Source: CAD feature listing. Evaluate the final solid. Frame: model axes, mm. Face numbers are marked on the shaded views. Coordinates: 2 decimals unless noted, no trailing zeros. Order: outer loops, then holes, each group sorted by start corner. A loop starts at its lowest first (then second) coordinate and runs counter-clockwise, first axis right, second up.
Autodesk Fusion 360 part; units mm, degrees
sketch "Sketch1" plane through (0, 0, 0) normal (0, 0, 1) x (1, 0, 0)
  line L0 (30, 30) -> (-30, 30)
  line L1 (-30, 30) -> (-30, -30)
  line L2 (-30, -30) -> (30, -30)
  line L3 (30, -30) -> (30, 30)
  line L4 (30, 30) -> (-30, -30) construction
  line L5 (-30, 30) -> (30, -30) construction
  circle A0 centre (-30, 30) radius 2.8
  circle A1 centre (30, 30) radius 2.8
  circle A2 centre (-30, -30) radius 2.8
  circle A3 centre (30, -30) radius 2.8
  line L6 (50, 50) -> (-50, 50)
  line L7 (-50, 50) -> (-50, -50)
  line L8 (-50, -50) -> (50, -50)
  line L9 (50, -50) -> (50, 50)
  line L10 (50, 50) -> (-50, -50) construction
  line L11 (-50, 50) -> (50, -50) construction
  line L12 (50, 50) -> (-50, 50)
  line L13 (-50, 50) -> (-50, 60)
  line L14 (-50, 60) -> (50, 60)
  line L15 (50, 60) -> (50, 50)
  line L16 (50, -50) -> (-50, -50)
  line L17 (-50, -50) -> (-50, -60)
  line L18 (-50, -60) -> (50, -60)
  line L19 (50, -60) -> (50, -50)
  circle A4 centre (-30, 30) radius 2
  circle A5 centre (30, 30) radius 2
  circle A6 centre (-30, -30) radius 2
  circle A7 centre (30, -30) radius 2
  dimension "d1" = 60
  dimension "d2" = 60
  dimension "d3" = 5.6
  dimension "d6" = 60
  dimension "d7" = -60
  dimension "d8" = 100
  dimension "d9" = 100
  dimension "d12" = 100
  dimension "d13" = 10
  dimension "d14" = 100
  dimension "d15" = 10
  dimension "d26" = 4
extrude "Extrude1" add sketch "Sketch1" along normal blind 10 contours L0 L1 L2 L3 A0 A1 A2 A3 | L6 L7 L8 L9 L12 L16 makes body 1
extrude "Extrude2" add sketch "Sketch1" along normal blind 110 contours L6 L12 L13 L14 L15 | L8 L16 L17 L18 L19 bodies 1
sketch "Sketch2" plane through (0, 0, 110) normal (0, 0, 1) x (1, 0, 0)
  line L0 (50, 60) -> (-50, 60)
  line L1 (-50, 60) -> (-50, 50)
  line L2 (-50, 50) -> (50, 50)
  line L3 (50, 50) -> (50, 60)
  circle A0 centre (-40, 55) radius 2.8
  line L4 (-50, 55) -> (50, 55)
  circle A1 centre (0, 55) radius 2.8
  circle A2 centre (40, 55) radius 2.8
  circle A3 centre (-40, -55) radius 2.8
  circle A4 centre (0, -55) radius 2.8
  circle A5 centre (40, -55) radius 2.8
  line L5 (-50, 60) -> (50, 60)
  line L6 (50, 60) -> (50, -60)
  line L7 (50, -60) -> (-50, -60)
  line L8 (-50, -60) -> (-50, 60)
  circle A6 centre (-40, 55) radius 2.25
  circle A7 centre (0, 55) radius 2.25
  circle A8 centre (40, 55) radius 2.25
  circle A9 centre (-40, -55) radius 2.25
  circle A10 centre (0, -55) radius 2.25
  circle A11 centre (40, -55) radius 2.25
  dimension "d18" = 5.6
  dimension "d19" = 10
  dimension "d22" = 40
  dimension "d23" = -110
  dimension "d30" = 120
  dimension "d31" = 100
  dimension "d32" = 4.5
extrude "Extrude3" cut sketch "Sketch2" against normal blind 8.1 contours L4 A2 A8 | L4 A2 A8 | A0 L4 A6 | A0 L4 A6 | L4 A8 | L4 A8 | L4 A6 | L4 A6 | L4 A1 A7 | L4 A1 A7 | L4 A7 | L4 A7 | A3 | A4 | A5 | A9 | A10 | A11 bodies 1
extrude "Extrude4" add sketch "Sketch1" against normal blind 1.9 from surface at 10 contours L0 L1 A0 A4 | L0 L1 A0 A4 | L0 L3 A1 A5 | L0 L3 A1 A5 | L1 L2 A2 A6 | L1 L2 A2 A6 | L2 L3 A3 A7 | L2 L3 A3 A7 bodies 1
extrude "Extrude5" add sketch "Sketch2" along normal blind 12 separate body contours L0 L1 L3 A0 L4 A1 A2 L5 L6 L8 | L1 L2 L3 A0 L4 A1 A2 L6 L8 | L2 L6 L7 L8 | L4 A2 A8 | L4 A2 A8 | A0 L4 A6 | A0 L4 A6 | L4 A1 A7 | L4 A1 A7 | A3 | A4 | A5 makes body 2
chamfer "Chamfer1" distance 5 angle 45 4 edges at (-50, 0, 0) (0, 60, 0) (50, 0, 0) (0, -60, 0) on bodies 1
hidden bodies 2
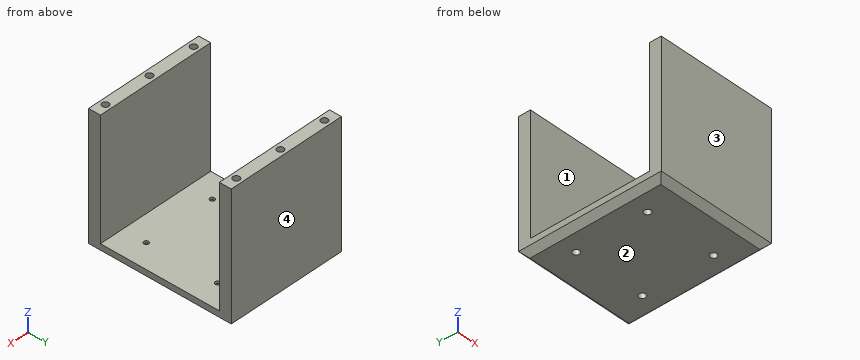
1. Section query C-C on x = 30. Return loops of the section in (y, z), plus the area to 3 significant figures.
Findings:
outline: (-60, 5) - (-55, 0) - (-32.8, 0) - (-32.8, 8.1) - (-32, 8.1) - (-32, 10) - (-50, 10) - (-50, 110) - (-60, 110) - close; (-28, 8.1) - (-27.2, 8.1) - (-27.2, 0) - (27.2, 0) - (27.2, 8.1) - (28, 8.1) - (28, 10) - (-28, 10) - close; (32, 8.1) - (32.8, 8.1) - (32.8, 0) - (55, 0) - (60, 5) - (60, 110) - (50, 110) - (50, 10) - (32, 10) - close
area: 3,070 mm2
2. Pin query (flat end, axial travel): P1, Ø5, axis at x = 14, y = -33.5, coming from the +Z side; P2, Ø3, axis at x = -41, y = -54.5, coming from the +Z side. Return the tip coordinate at first contact, or that it passes through.
Findings:
P1: stops at z = 10
P2: stops at z = 101.9
3. Draft query along Y for the marked faces 1, 2, 3 and 4. Return one class per face: released by +Y, released by -Y, zero draft, split by the parting line, or undercut.
Findings:
face 1: undercut
face 2: zero draft
face 3: released by -Y
face 4: released by +Y
4. Section query D-D on x = 0. Return loops of the section in (y, z), plus the area to 3 significant figures.
Findings:
outline: (-60, 5) - (-55, 0) - (55, 0) - (60, 5) - (60, 110) - (57.8, 110) - (57.8, 101.9) - (52.2, 101.9) - (52.2, 110) - (50, 110) - (50, 10) - (-50, 10) - (-50, 110) - (-52.2, 110) - (-52.2, 101.9) - (-57.8, 101.9) - (-57.8, 110) - (-60, 110) - close
area: 3,080 mm2
5. Section query A-A on z = 68. Return loops of the section in (x, y).
Findings:
outline: (-50, -60) - (50, -60) - (50, -50) - (-50, -50) - close; (-50, 50) - (50, 50) - (50, 60) - (-50, 60) - close
6. Ray query, line 1 (Y direction, x = -40, z = 105); line 2 (X direction, y = 55, z = 108); line 3 (Y direction, x = 30, z = 8). Return the intervals inside material, ascending.
Findings:
line 1: y = -60 to -57.8, -52.2 to -50, 50 to 52.2, 57.8 to 60
line 2: x = -50 to -42.8, -37.2 to -2.8, 2.8 to 37.2, 42.8 to 50
line 3: y = -60 to -32.8, -27.2 to 27.2, 32.8 to 60
7. Section query B-B on y = -30. Return loops of the section in (x, z), plus the area to 3 significant figures.
Findings:
outline: (-50, 5) - (-45, 0) - (-32.8, 0) - (-32.8, 8.1) - (-32, 8.1) - (-32, 10) - (-50, 10) - close; (-28, 8.1) - (-27.2, 8.1) - (-27.2, 0) - (27.2, 0) - (27.2, 8.1) - (28, 8.1) - (28, 10) - (-28, 10) - close; (32, 8.1) - (32.8, 8.1) - (32.8, 0) - (45, 0) - (50, 5) - (50, 10) - (32, 10) - close
area: 869 mm2
